```python
from build123d import *

# Parameters (mm, degrees)
F0_W     = 533.4
F0_H     = 635
F1_DEPTH = 50.8
F2_W     = 533.4
F2_H     = 127
F3_DEPTH = 508
F4_R     = 76.2
F5_DEPTH = 406.4


with BuildPart() as f1:
    # F0 (on Top) → F1 (new body)
    with BuildSketch(Plane.XY):
        with Locations((266.7, 317.5)):
            Rectangle(F0_W, F0_H)
    extrude(amount=F1_DEPTH)

    # F2 (on face) → F3 (join)
    with BuildSketch(Plane.XY.offset(50.8)):
        with Locations((266.7, 63.5)):
            Rectangle(F2_W, F2_H)
    extrude(amount=F3_DEPTH)

    # F4 (on face) → F5 (join)
    with BuildSketch(Plane(origin=(0, 0, 0), x_dir=(1, 0, 0), z_dir=(0, 0, -1))):
        with Locations((266.7, -317.5)):
            Circle(F4_R)
    extrude(amount=F5_DEPTH)


solid = f1.part
```
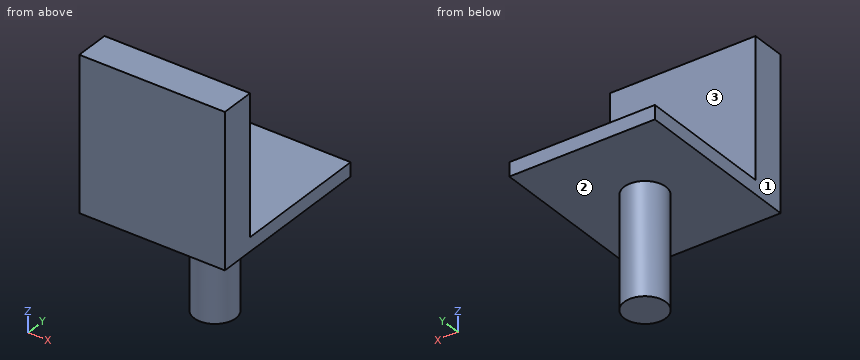
The listing builds one solid part. Answer for the finished solid, in the listing's coordinates (mm). Face numbers are marked on the shaded views. A direction names the side the tool comes from. Round coordinates to 2 decimals unless told otherwise and drop trailing zeros. Loops run counter-clockwise (first coordinate to the right, second up) from the corner with the lowest first, then second, coordinate; pieces in that order, holes last. Notation, with made-up numbers: (87, -6) - (130, -6) arc R20 ccw to (130, 0) - close; hole circle Ø6 at (46, 42.25). An arc over 180 degrees is marked (long way). Return JSON: item names as keys, results as strings. Group by question number.
1. Consider probe 1 along Z at (x, y) = (354, 154.5); probe 2 along Z at (x, y) = (324, 323); probe 3 along Y at (x, z) = (201.5, 79). Determine where each line is inside the solid, lowest interval first.
2. The part is cut by section C-C on z = 123. Determine the outline of the cut face in (x, y).
3. Which of the six approach directions +Z, -Z, +X, -X, +Y, -Y give full straight-line access (tool end or side, diameter ignored) to the marked faces 1, 2 and 3?
4. The part is cut by section D-D on x = 42. Determine the outline of the cut face in (y, z), then the cut area to 3 significant figures.
5. The part is cut by section A-A on x = 266.7. Determine the outline of the cut face in (y, z), then the cut area to 3 significant figures.
6. Each of these flat-tipped pins is pushed along its axis until it touches: P1, Ø12, axis at x = 224, z = -17.5, coming from the -Y side; P2, Ø8, axis at y = 307.5, z = -225, coming from the -X side; P3, Ø1, axis at x = 157.5, z = 333, coming from the -Y side; P4, Ø2, axis at x = 233.5, y = 491.5, coming from the +Z side. Where does it stop, or does it pass through?
7. The part is cut by section B-B on y = 317.5. Determine the outline of the cut face in (x, z).
Resolved:
{
 "1": {"probe 1": "z = 0 to 50.8", "probe 2": "z = -406.4 to 50.8", "probe 3": "y = 0 to 127"},
 "2": {"outline": "(0, 0) - (533.4, 0) - (533.4, 127) - (0, 127) - close"},
 "3": {"face 1": "+Z, -Z, -X, +Y, -Y", "face 2": "-Z", "face 3": "+Z, +X, -X, +Y"},
 "4": {"outline": "(0, 0) - (635, 0) - (635, 50.8) - (127, 50.8) - (127, 558.8) - (0, 558.8) - close", "area": "96,800 mm²"},
 "5": {"outline": "(0, 0) - (241.3, 0) - (241.3, -406.4) - (393.7, -406.4) - (393.7, 0) - (635, 0) - (635, 50.8) - (127, 50.8) - (127, 558.8) - (0, 558.8) - close", "area": "159,000 mm²"},
 "6": {"P1": "stops at y = 250.72", "P2": "stops at x = 190.74", "P3": "stops at y = 0", "P4": "stops at z = 50.8"},
 "7": {"outline": "(0, 0) - (190.5, 0) - (190.5, -406.4) - (342.9, -406.4) - (342.9, 0) - (533.4, 0) - (533.4, 50.8) - (0, 50.8) - close"}
}
